The listing builds one solid part. Answer for the finished solid, in the listing's coordinates (mm). A direction names the side the tool comes from. Round coordinates to 2 decimals unless told otherwise and drop trailing zeros. Write each loop counter-clockwise with the first axis right and the second up, starting at its lowest first coordinate (ties: lowest second). Pieces come first, ordered by that corner, then holes. Notation, with made-up numbers: M 31.25,39.5 L 45.25,39.5 A16 cw 45.25,65.5 Z; hole C 68,16.25 d9. An arc over 180 degrees is marked long. Write each question's results on one line, items separated by ' | '.
from build123d import *

# Parameters (mm, degrees)
SKETCH1_W           = 30
SKETCH1_H           = 30
BOSS_EXTRUDE2_DEPTH = 5
SKETCH3_R           = 1.02617269
CUT_EXTRUDE1_DEPTH  = 5
SKETCH4_W           = 10
SKETCH4_H           = 30
BOSS_EXTRUDE3_DEPTH = 30
SKETCH5_R           = 2.55
CUT_EXTRUDE2_DEPTH  = 30
FILLET1_R           = 10
FILLET2_R           = 10
FILLET4_R           = 3
FILLET5_R           = 3


with BuildPart() as part:
    # Sketch1 → Boss-Extrude2 (new body)
    with BuildSketch(Plane.XY):
        Rectangle(SKETCH1_W, SKETCH1_H)
    extrude(amount=BOSS_EXTRUDE2_DEPTH)

    # Sketch3 → Cut-Extrude1 (cut)
    with BuildSketch(Plane.XY.offset(5)):
        with Locations((-11.9939671, 11.375061325)):
            Circle(SKETCH3_R)
        with Locations((11.375061325, 11.9939671)):
            Circle(SKETCH3_R)
        with Locations((11.9939671, -11.375061325)):
            Circle(SKETCH3_R)
        with Locations((-11.375061325, -11.9939671)):
            Circle(SKETCH3_R)
    extrude(amount=-CUT_EXTRUDE1_DEPTH, mode=Mode.SUBTRACT)

    # Sketch4 → Boss-Extrude3 (add)
    with BuildSketch(Plane.XY.offset(5)):
        Rectangle(SKETCH4_W, SKETCH4_H)
    extrude(amount=BOSS_EXTRUDE3_DEPTH)

    # Sketch5 → Cut-Extrude2 (cut)
    with BuildSketch(Plane(origin=(5, 0, 0), x_dir=(0, 0, -1), z_dir=(1, 0, 0))):
        with Locations((-22, 0)):
            Circle(SKETCH5_R)
    extrude(amount=-CUT_EXTRUDE2_DEPTH, mode=Mode.SUBTRACT)

    # Fillet1
    fillet1_edges = [part.edges().sort_by_distance(p)[0] for p in [
        (0, -15, 35),
    ]]
    fillet(fillet1_edges, radius=FILLET1_R)

    # Fillet2
    fillet2_edges = [part.edges().sort_by_distance(p)[0] for p in [
        (0, 15, 35),
    ]]
    fillet(fillet2_edges, radius=FILLET2_R)

    # Fillet4
    fillet4_edges = [part.edges().sort_by_distance(p)[0] for p in [
        (5, 0, 5),
    ]]
    fillet(fillet4_edges, radius=FILLET4_R)

    # Fillet5
    fillet5_edges = [part.edges().sort_by_distance(p)[0] for p in [
        (-5, 0, 5),
    ]]
    fillet(fillet5_edges, radius=FILLET5_R)


solid = part.part
1) Section C-C (x = 2.75) is taken. Determine the outline of the cut face in (y, z), then the cut area to 3 significant figures.
Return value:
outline: M -15,0 L 15,0 L 15,25 A10 ccw 5,35 L -5,35 A10 ccw -15,25 Z; hole C 0,22 d5.1 | area: 987 mm²
2) The mould has two halves that part along X. Classify faces 1 (the face through (0, 15, 10)), 2 (the face through (-5, 0, 18)), 3 (the face through (-12.216, 10.373, 2.535)): +X half, -X half, draft (parallel to the pull), parting line (faces both ways), or undercut.
Return value:
face 1: draft | face 2: -X half | face 3: undercut
3) Each of these flat-tipped pins is pushed along its axis until it touches: pin 1 (6 mm diameter, centred on y = -1.5, z = 28, fed in from +X); pin 2 (3.5 mm diameter, centred on x = -11.38, y = -11.99, fed in from +Z); pin 3 (8 mm diameter, centred on y = 7.5, z = 20.5, fed in from -X); pin 4 (2.5 mm diameter, centred on x = -11.99, y = 11.38, fed in from -Z). Where does it stop, or does it pass through?
Return value:
pin 1: x = 5 | pin 2: z = 5 | pin 3: x = -5 | pin 4: z = 0
4) Find the intervals of material crossed by line 1 (Y direction, x = -0.75, z = 22); line 2 (Z direction, x = 11, y = -4.5); line 3 (X direction, y = -11, z = 26), in increasing order.
Return value:
line 1: -15 to -2.55, 2.55 to 15 | line 2: 0 to 5 | line 3: -5 to 5
5) Section A-A (y = 0) is taken. Determine the outline of the cut face in (x, z).
Return value:
outline: M -15,0 L 15,0 L 15,5 L 8,5 A3 cw 5,8 L 5,19.45 L -5,19.45 L -5,8 A3 cw -8,5 L -15,5 Z; M -5,24.55 L 5,24.55 L 5,35 L -5,35 Z
6) A tool of negligible diameter and unlimited length cuts with its end or side. For faces 4 (the face through (-12, 0, 5)), 5 (the face through (11, 0, 5)), 6 (the face through (-15, 0, 2)), from which of +Z, -Z, +X, -X, +Y, -Y can it reach the whole face along a straight path? Write none if from no direction.
Return value:
face 4: +Z, -X, +Y, -Y | face 5: +Z, +X, +Y, -Y | face 6: +Z, -Z, -X, +Y, -Y
7) Section D-D (y = -6) is taken. Determine the outline of the cut face in (x, z).
Return value:
outline: M -15,0 L 15,0 L 15,5 L 8,5 A3 cw 5,8 L 5,34.95 L -5,34.95 L -5,8 A3 cw -8,5 L -15,5 Z
8) Section B-B (z = 22) is taken. Determine the outline of the cut face in (x, y), then the cut area to 3 significant figures.
Return value:
outline: M -5,-15 L 5,-15 L 5,-2.55 L -5,-2.55 Z; M -5,2.55 L 5,2.55 L 5,15 L -5,15 Z | area: 249 mm²
